The model under review builds one solid part; all positions refer to its coordinate system, in mm. Round coordinates to 2 decimals unless told otherwise and drop trailing zeros. Write each loop counter-clockwise with the first axis right and the second up, starting at its lowest first coordinate (ties: lowest second). Pieces come first, ordered by that corner, then holes. Notation, with made-up numbers: M 48,-6 L 73,-6 A30 cw 73,17 Z; hole C 0,-31.75 d4. An arc over 180 degrees is marked long. Write item = value, one per line. Start each with the question number.
Item 1: Take a section at C-C, the plane y = -6.25. Give the boundary of the cut face in (x, z), plus the area to 3 significant figures.
Item 2: The part is to be moulded in two halves that separate along X. For faces 1 (the flat face through (-40, -4, 2)), 2 (the cylindrical face through (1.802, -3.944, 5.723)), 3 (the flat face through (-1, 0, -9)), say which applies: +X half, -X half, draft (parallel to the pull), parting line (faces both ways), or undercut.
Item 3: To check wall thickness, follow line 1 along X through (y, z) = (-2.5, 0); line 2 along X through (y, z) = (-0.5, 4); line 3 along Z through (x, y) = (2, -2). State the ranges of each line that lie inside material, in increasing order.
Item 4: Take a section at A-A, the plane z = 0. Give the boundary of the cut face in (x, y).
Item 5: Take a section at B-B, the plane x = 0. Give the boundary of the cut face in (y, z), plus the area to 3 significant figures.
Item 6: For pin 1 Ø7 at (x, z) = (0, 0) entering from +Y; pin 2 Ø10 at (x, z) = (-10.5, 11) entering from +Y, all flat-tipped, find the tip position at first contact; note any pin that passes through.
from build123d import *

# Parameters (mm, degrees)
SKETCH1_W          = 80
SKETCH1_H          = 40
BASE_FLANGE1_DEPTH = 8
SKETCH6_R          = 6
CUT_EXTRUDE1_DEPTH = 10
FILLET1_R          = 3.74


# Sheet-metal steps are written as plain solids
with BuildPart() as part:
    # Sketch1 → Base-Flange1 (new body)
    with BuildSketch(Plane(origin=(0, 0, 0), x_dir=(1, 0, 0), z_dir=(0, 1, 0))):
        Rectangle(SKETCH1_W, SKETCH1_H)
    extrude(amount=-BASE_FLANGE1_DEPTH)

    # Sketch6 → Cut-Extrude1 (cut)
    with BuildSketch(Plane(origin=(0, 0, 0), x_dir=(1, 0, 0), z_dir=(0, 1, 0))):
        with Locations(Location((0, 0, 0), (0, 0, 270))):
            Circle(SKETCH6_R)
    extrude(amount=-CUT_EXTRUDE1_DEPTH, mode=Mode.SUBTRACT)

    # Fillet1
    fillet1_edges = [part.edges().sort_by_distance(p)[0] for p in [
        (-40, -4, -20),
        (40, -4, -20),
    ]]
    fillet(fillet1_edges, radius=FILLET1_R)


solid = part.part
Response values:
q1.outline = M -40,-16.26 A3.74 ccw -36.26,-20 L 36.26,-20 A3.74 ccw 40,-16.26 L 40,20 L -40,20 Z; hole C 0,0 d12
q1.area = 3,080 mm2
q2.face_1 = -X half
q2.face_2 = undercut
q2.face_3 = draft
q3.line_1 = -40 to -6, 6 to 40
q3.line_2 = -40 to -4.47, 4.47 to 40
q3.line_3 = -20 to -5.66, 5.66 to 20
q4.outline = M -40,-8 L -6,-8 L -6,0 L -40,0 Z; M 6,-8 L 40,-8 L 40,0 L 6,0 Z
q5.outline = M -8,-20 L 0,-20 L 0,-6 L -8,-6 Z; M -8,6 L 0,6 L 0,20 L -8,20 Z
q5.area = 224 mm2
q6.pin_1 = through
q6.pin_2 = 0
